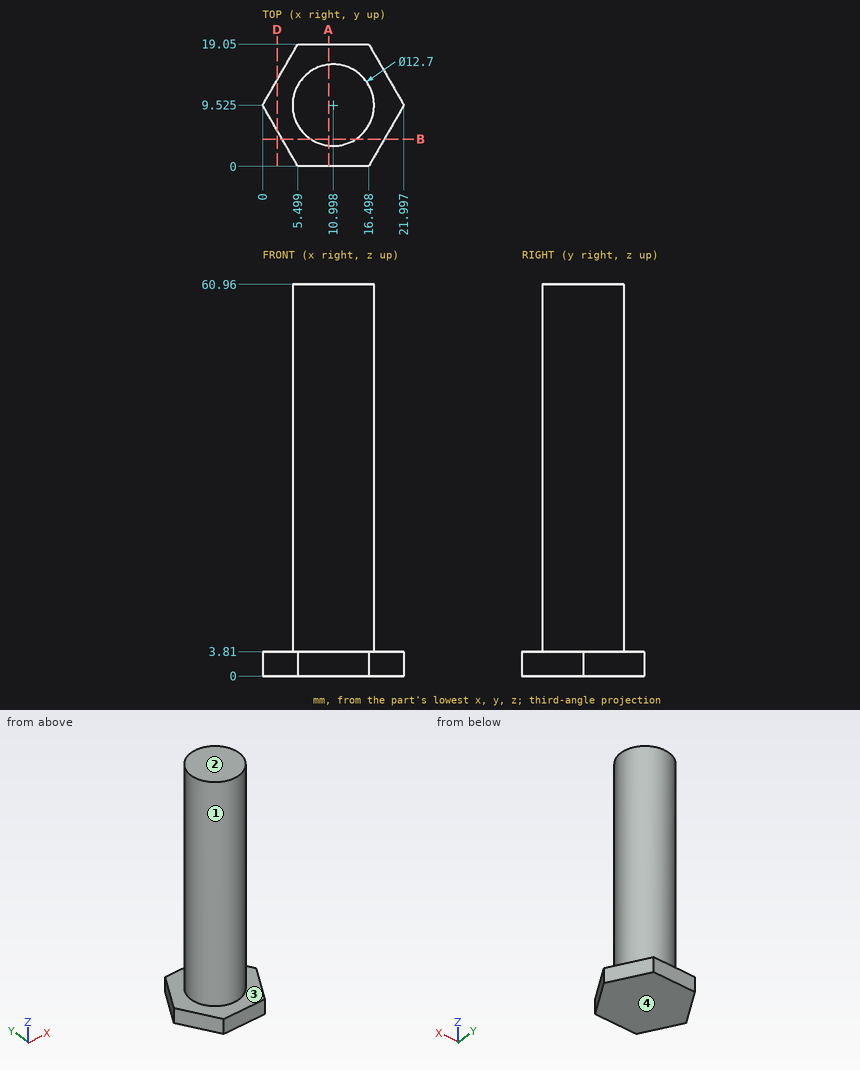
Part print with two shaded views. Sizes in mm from the minimum x, y, z corner. A direction names the side the tool comes from. Give positions to 0.01 mm unless a question says otherwise; leave off trailing zeros. Order: outer loops, then holes, each group sorted by start corner. A loop starts at its lowest first (then second) coordinate and runs counter-clockwise, first axis right, second up. Notation, with made-up numbers: M 19.5,77.5 L 57.5,77.5 A30 cw 57.5,100.5 Z; hole C 77.5,89.5 d3. An arc over 180 degrees is marked long. Write item = value, one per line.
Q1. Cut at A-A, the plane x = 10.25. List the corners of the cut face in (y, z).
Derived:
outline = M 0,0 L 19.05,0 L 19.05,3.81 L 15.83,3.81 L 15.83,60.96 L 3.22,60.96 L 3.22,3.81 L 0,3.81 Z
Q2. Drill centre lines: line 1 (X direction, y = 9.5, z = 57.5); line 2 (Z direction, x = 15.75, y = 17); line 3 (Y direction, x = 6.75, z = 42.5) (1 decimal). Where is each one in solid material? Low to high. Write a range as [from, to].
Derived:
line_1 = [4.65, 17.35]
line_2 = [0, 3.81]
line_3 = [4.8, 14.2]
Q3. Two-plate mould, pull along X, no slides. Class the marked faces 1 and 2: pulls with the +X half, pulls with the -X half, needs draft (parallel to the pull), parting line crosses it, or undercut.
Derived:
face_1 = parting line crosses it
face_2 = needs draft
Q4. Cut at D-D, the plane x = 2.25. List the corners of the cut face in (y, z), then the cut area to 3 significant figures.
Derived:
outline = M 5.63,0 L 13.42,0 L 13.42,3.81 L 5.63,3.81 Z
area = 29.7 mm2
Q5. Cut at B-B, the plane y = 4.25. List the corners of the cut face in (x, z) (1 decimal).
Derived:
outline = M 3,0 L 19,0 L 19,3.8 L 14.5,3.8 L 14.5,61 L 7.5,61 L 7.5,3.8 L 3,3.8 Z
Q6. Tool access for the marked faces 3 and 4: list every direction of +Z, -Z, +X, -X, +Y, -Y with a clear straight run to the whole face (end or side of a thin tool).
Derived:
face_3 = +Z
face_4 = -Z, +X, -X, +Y, -Y
Q7. Flat gauge pins, fed straight in: pin 1 (4 mm diameter, centred on y = 2, z = 18.5, fed in from +X); pin 2 (5 mm diameter, centred on y = 16, z = 28.5, fed in from -X) (1 decimal); pin 3 (3 mm diameter, centred on x = 18, y = 2.5, fed in from +Z). Where does each tip first touch, or does it go through?
Derived:
pin_1 = 14.13
pin_2 = 6
pin_3 = 3.81
